Part model, mm, in its own coordinate system. Face numbers are marked on the shaded views. Give positions to 0.01 mm unless a question says otherwise; leave off trailing zeros. Order: outer loops, then holes, each group sorted by start corner. A loop starts at its lowest first (then second) coordinate and runs counter-clockwise, first axis right, second up. Notation, with made-up numbers: M 83.5,-9.5 L 99.5,-9.5 A38 cw 99.5,28.5 Z; hole C 23.25,-15 d3. An arc over 180 degrees is marked long. Answer as a JSON object with one key per item and string values.
from build123d import *


with BuildPart() as part:
    # Sketch2 one side → Revolve-Thin1 (revolve)
    with BuildSketch(Plane.XY, mode=Mode.PRIVATE) as revolve_thin1_sk:
        Polygon((-325.5, 1707.83763204), (-325.5, 2040), (-367.75, 2040), (-367.75, 2015), (-352.5, 2015), (-352.5, 1984.235457461), (-369.75, 1949.635457461), (-369.75, 1707.83763204), align=None)
        Polygon((-366.75, 2039), (-326.5, 2039), (-326.5, 1708.83763204), (-368.75, 1708.83763204), (-368.75, 1949.4), (-351.5, 1984), (-351.5, 2016), (-366.75, 2016), align=None, mode=Mode.SUBTRACT)
    revolve(revolve_thin1_sk.sketch.rotate(Axis((0, 1764, 0), (0, 1, 0)), 270), axis=Axis((0, 1764, 0), (0, 1, 0)))  # turned: the seam where the file's is


solid = part.part
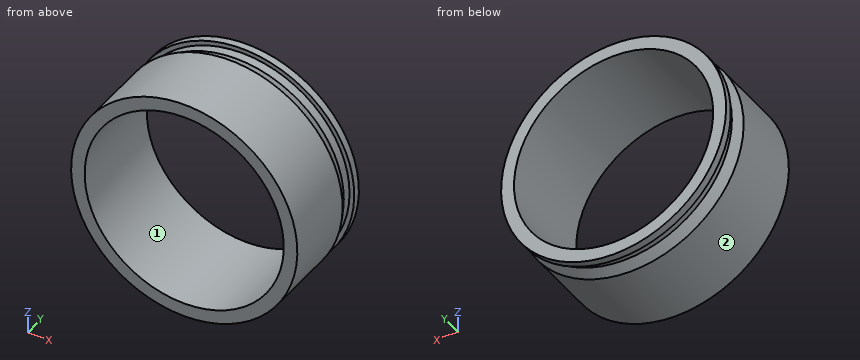
1. Cut at C-C on y = 1825.5. Give the cut face in (x, z), plus the area to 3 significant figures.
Worked answers:
{"outline": "C 0,0 d739.5; C 0,0 d653; hole C 0,0 d737.5; hole C 0,0 d651", "area": "4,370 mm^2"}
2. Cut at A-A on x = 0. State how many separate pieces and enclosed holes the cut face has, plus the area to 3 significant figures.
Worked answers:
{"separate pieces": "2", "enclosed holes": "2", "area": "1,530 mm^2"}
3. Two-plate mould, pull along X, no slides. Class the marked faces 1 and 2: +X half, -X half, draft (parallel to the pull), parting line (faces both ways), or undercut.
Worked answers:
{"face 1": "undercut", "face 2": "parting line"}
4. Probe line 1 along X through (y, z) = (1855.5, 0); line 2 along X through (y, z) = (2003, 0); line 3 along Z through (x, y) = (-165, 2019). List the from-to ranges inside material, lowest first.
Worked answers:
{"line 1": "x = -369.75 to -368.75, -326.5 to -325.5, 325.5 to 326.5, 368.75 to 369.75", "line 2": "x = -352.5 to -351.5, -326.5 to -325.5, 325.5 to 326.5, 351.5 to 352.5", "line 3": "z = -328.66 to -327.54, -281.74 to -280.58, 280.58 to 281.74, 327.54 to 328.66"}
5. Pin check, flat tips, straight feed: P1, Ø12, axis at y = 1752, z = 148.5, coming from the +X side; P2, Ø12, axis at y = 1973.5, z = -65, coming from the +X side; P3, Ø5, axis at x = -123, y = 1975, coming from the -Z side. Stop position of each tip, or through.
Worked answers:
{"P1": "stops at x = 341.19", "P2": "stops at x = 355.13", "P3": "stops at z = -336.86"}
